Source: CAD feature listing. Evaluate the final solid. Frame: model axes, mm. A direction names the side the tool comes from. Coordinates: 2 decimals unless noted, no trailing zeros. Order: outer loops, then holes, each group sorted by start corner. A loop starts at its lowest first (then second) coordinate and runs counter-clockwise, first axis right, second up.
```python
from build123d import *

# Parameters (mm, degrees)
F0_R     = 2.032
F1_DEPTH = 5.715
F2_W     = 83.82
F2_H     = 12.7
F2_R     = 2.0955
F2_R_2   = 1.5875
F2_R_3   = 2.296673
F3_DEPTH = 2.54


with BuildPart() as f1:
    # F0 (on Top) → F1 (new body)
    with BuildSketch(Plane.XY):
        with BuildLine():
            Line((-15.475456, 42.854359), (-5.369036, -55.16359))
            ThreePointArc((-5.369036, -55.16359), (0, -60.0075), (5.369036, -55.16359))
            Line((5.369036, -55.16359), (15.475456, 42.854359))
            ThreePointArc((15.475456, 42.854359), (0, 60.0075), (-15.475456, 42.854359))
        make_face()
        with Locations((0, -54.61)):
            Circle(F0_R, mode=Mode.SUBTRACT)
        with Locations((-5.08, 44.45)):
            Circle(F0_R, mode=Mode.SUBTRACT)
        with Locations((5.08, 44.45)):
            Circle(F0_R, mode=Mode.SUBTRACT)
    extrude(amount=-F1_DEPTH)

    # F2 (on Right) → F3 (join, symmetric)
    with BuildSketch(Plane.YZ):
        with Locations((-5.986101, 6.35)):
            Rectangle(F2_W, F2_H)
        with Locations((-41.516703, 6.35)):
            Circle(F2_R, mode=Mode.SUBTRACT)
        with Locations((-30.626114, 6.35)):
            Circle(F2_R_2, mode=Mode.SUBTRACT)
        with Locations((29.573899, 6.35)):
            Circle(F2_R_3, mode=Mode.SUBTRACT)
    extrude(amount=F3_DEPTH, both=True)


solid = f1.part
```
Q1. Pin query (flat end, axial travel): P1, Ø2.5, axis at x = 1.5, z = 5, coming from the +Y side; P2, Ø3.5, axis at x = -5.08, y = 44.45, coming from the +Z side; P3, Ø4, axis at y = -1, z = 8.5, coming from the -X side; P4, Ø5.5, axis at x = -0.5, z = 6, coming from the -Y side. Return the tip coordinate at first contact, or that it passes through.
Solutions:
P1: stops at y = 35.92
P2: passes through
P3: stops at x = -2.54
P4: stops at y = -47.9
Q2. Pull-direction query (Z, two-part tool) for faces 1 (the cylindrical face through (-0.04, -39.52, 6.98)), 2 (the flat face through (0, 35.924, 6)), 3 (the flat face through (0, -7, 12.7)), 4 (the cylindrical face through (-0.04, 27.28, 6.45)); classes: pulls with the +Z half, pulls with the -Z half, needs draft (parallel to the pull), parting line crosses it, or undercut.
Solutions:
face 1: undercut
face 2: needs draft
face 3: pulls with the +Z half
face 4: undercut
Q3. Material intervals for line 1 along Y through (x, z) = (1.5, 3); line 2 along X through (y, z) = (-44, 8); line 3 along Z through (x, y) = (-4, -9) (3 decimals), sorted ascending.
Solutions:
line 1: y = -47.9 to 35.92
line 2: x = -2.54 to 2.54
line 3: z = -5.715 to 0
Q4. Section query C-C on z = 10.75. Output: boundary loops of the cut face in (x, y), plus the area to 3 significant figures.
Solutions:
outline: (-2.54, -47.9) - (2.54, -47.9) - (2.54, 35.92) - (-2.54, 35.92) - close
area: 426 mm2
Q5. Section query A-A on x = 0. Give the number of separate pieces and of enclosed holes in the cut face, plus the area to 3 significant figures.
Solutions:
separate pieces: 2
enclosed holes: 3
area: 1,690 mm2
Q6. Section query D-D on y = -28. Output: boundary loops of the cut face in (x, z) (3 decimals).
Solutions:
outline: (-8.17, -5.715) - (8.17, -5.715) - (8.17, 0) - (2.54, 0) - (2.54, 12.7) - (-2.54, 12.7) - (-2.54, 0) - (-8.17, 0) - close
Q7. Set-up query: faces 5 (the flat face through (2.54, -7, 6)), 6 (the flat face through (0, -47.896, 6)), 7 (the flat face through (-2.54, -7, 6)), 8 (the cylindrical face through (-0.111, -60.006, -2.817)). Return all of +Z, -Z, +X, -X, +Y, -Y with unobstructed straight access to the full face (end or side cutting, diameter ignored); none if empty.
Solutions:
face 5: +Z, +X, +Y, -Y
face 6: +Z, +X, -X, -Y
face 7: +Z, -X, +Y, -Y
face 8: +Z, -Z, -Y
Q8. Section query B-B on y = 44.45. Output: boundary loops of the cut face in (x, z) (1 decimal), plus the area to 3 significant figures.
Solutions:
outline: (-15.6, -5.7) - (-7.1, -5.7) - (-7.1, 0) - (-15.6, 0) - close; (-3, -5.7) - (3, -5.7) - (3, 0) - (-3, 0) - close; (7.1, -5.7) - (15.6, -5.7) - (15.6, 0) - (7.1, 0) - close
area: 131 mm2
